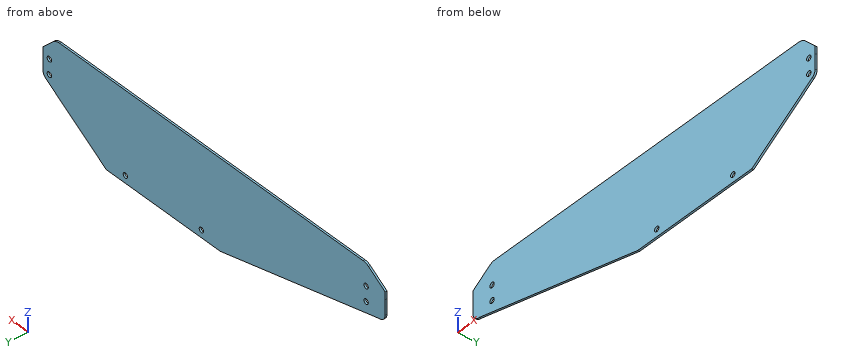
Autodesk Inventor part; units mm, degrees
ref_plane "YZ Plane" through (0, 0, 0) normal (1, 0, 0) x (0, 1, 0)
ref_plane "XZ Plane" through (0, 0, 0) normal (0, 1, 0) x (-1, 0, 0)
ref_plane "XY Plane" through (0, 0, 0) normal (0, 0, 1) x (1, 0, 0)
sketch "main" plane through (0, 0, 0) normal (0, 0, 1) x (1, 0, 0)
  circle A0 centre (45.9011, -170.4057) radius 2.1844
  circle A1 centre (58.6011, -170.4057) radius 2.1844
  arc A2 (39.5511, -183.1057) -> (45.9011, -189.4557) centre (45.9011, -183.1057) ccw
  line L0 (45.9011, -189.4557) -> (58.6011, -189.4557)
  line L1 (39.5511, -183.1057) -> (1.4511, -24.3557)
  arc A3 (76.0514, -172.8053) -> (77.6511, -167.5218) centre (68.1261, -167.5218) ccw
  line L2 (64.9511, -189.4557) -> (76.0514, -172.8053)
  line L3 (58.6011, -189.4557) -> (64.9511, -189.4557)
  circle A4 centre (45.9011, 147.0943) radius 2.1844
  circle A5 centre (58.6011, 147.0943) radius 2.1844
  circle A6 centre (7.8011, -5.3057) radius 2.1844
  circle A7 centre (7.8011, 70.8943) radius 2.1844
  line L4 (77.6511, -167.5218) -> (77.6511, 136.7989)
  line L5 (1.4511, -24.3557) -> (1.4511, 89.9443)
  arc A8 (77.6511, 136.7989) -> (74.8613, 143.5341) centre (68.1261, 136.7989) ccw
  line L6 (74.8613, 143.5341) -> (64.9511, 153.4443)
  line L7 (64.9511, 153.4443) -> (58.6011, 153.4443)
  line L8 (45.9011, 153.4443) -> (58.6011, 153.4443)
  arc A9 (45.9011, 153.4443) -> (40.5661, 150.5382) centre (45.9011, 147.0943) ccw
  line L9 (1.4511, 89.9443) -> (40.5661, 150.5382)
  point P0 (53.0582, -9.4982)
  point P1 (77.6511, -170.4057)
  point P2 (77.6511, -189.4557)
  point P3 (77.6511, 140.7443)
  point P4 (77.6511, 153.4443)
  dimension "d0" = 19.05
  dimension "d1" = 12.7
  dimension "d2" = 19.05
  dimension "d3" = 12.7
  dimension "d4" = 12.7
  dimension "d5" = 19.05
  dimension "d6" = 9.525
sketch "Sketch1" plane through (0, 0, 0) normal (0, 1, 0) x (-1, 0, 0)
  circle A0 centre (165.1067, 38.0709) radius 2.1844
  circle A1 centre (165.109, 50.7709) radius 2.1844
  arc A2 (177.8056, 31.7187) -> (184.1567, 38.0675) centre (177.8067, 38.0687) ccw
  line L0 (184.1567, 38.0675) -> (184.159, 50.7675)
  line L1 (177.8056, 31.7187) -> (19.0489, -6.3534)
  arc A3 (167.5116, 68.2207) -> (162.2284, 69.8214) centre (162.2267, 60.2964) ccw
  line L2 (184.1601, 57.1175) -> (167.5116, 68.2207)
  line L3 (184.159, 50.7675) -> (184.1601, 57.1175)
  circle A4 centre (-152.3933, 38.1269) radius 2.1844
  circle A5 centre (-152.391, 50.8269) radius 2.1844
  circle A6 centre (0, 0) radius 2.1844
  circle A7 centre (-76.2, 0.0134) radius 2.1844
  line L4 (162.2284, 69.8214) -> (-142.0923, 69.8751)
  line L5 (19.0489, -6.3534) -> (-95.2511, -6.3332)
  arc A8 (-142.0923, 69.8751) -> (-148.828, 67.0864) centre (-142.094, 60.3501) ccw
  line L6 (-148.828, 67.0864) -> (-158.7399, 57.178)
  line L7 (-158.7399, 57.178) -> (-158.741, 50.828)
  line L8 (-158.7433, 38.128) -> (-158.741, 50.828)
  arc A9 (-158.7433, 38.128) -> (-155.8381, 32.7925) centre (-152.3933, 38.1269) ccw
  line L9 (-95.2511, -6.3332) -> (-155.8381, 32.7925)
  point P0 (0, 0)
extrude "Extrusion1" add sketch "Sketch1" along normal blind 1.5875
properties part number "skirt" material "Acetal Resin, White"
Read the model definition and answer for the solid it produces. Units are mm, in the model's axes. Coordinates: 2 decimals unless noted, no trailing zeros. Order: outer loops, then holes, each group sorted by start corner. A loop starts at its lowest first (then second) coordinate and runs counter-clockwise, first axis right, second up. Notation, with made-up numbers: (40.25, -25.75) -> (89.25, -25.75) arc R27 cw to (89.25, 6.25) -> close; hole circle Ø6 at (-24, 58.5). An arc over 180 degrees is marked (long way). Answer as a JSON object with one key per item and string values.
1) A cutting plane is placed at A-A, the plane y = 1.3. Determine the outline of the cut face in (x, z).
Model answer:
{"outline": "(-184.16, 38.07) arc R6.35 ccw to (-177.81, 31.72) -> (-19.05, -6.35) -> (95.25, -6.33) -> (155.84, 32.79) arc R6.35 ccw to (158.74, 38.13) -> (158.74, 50.83) -> (158.74, 57.18) -> (148.83, 67.09) arc R9.52 ccw to (142.09, 69.88) -> (-162.23, 69.82) arc R9.53 ccw to (-167.51, 68.22) -> (-184.16, 57.12) -> (-184.16, 50.77) -> close; hole circle Ø4.37 at (-165.11, 38.07); hole circle Ø4.37 at (-165.11, 50.77); hole circle Ø4.37 at (0, 0); hole circle Ø4.37 at (76.2, 0.01); hole circle Ø4.37 at (152.39, 38.13); hole circle Ø4.37 at (152.39, 50.83)"}
2) Consider line 1 along Z through (x, y) = (0, 0.9); line 2 along X through (y, z) = (0.8, 36.5); line 3 along X through (y, z) = (1.05, 47). Determine where each line is inside the solid, lowest interval first. Write a range as from..to.
Model answer:
{"line 1": "z = -6.35..-2.18, 2.18..69.85", "line 2": "x = -183.96..-166.62, -163.59..150.94, 153.85..158.53", "line 3": "x = -184.16..158.74"}
3) Each of these flat-tipped pins is pushed along its axis until it touches: pin 1 (4 mm diameter, centred on x = 0, z = 0, fed in from -Y); pin 2 (0.5 mm diameter, centred on y = 1, z = 43.5, fed in from -X). Where does it stop, or does it pass through?
Model answer:
{"pin 1": "passes through", "pin 2": "stops at x = -184.16"}
